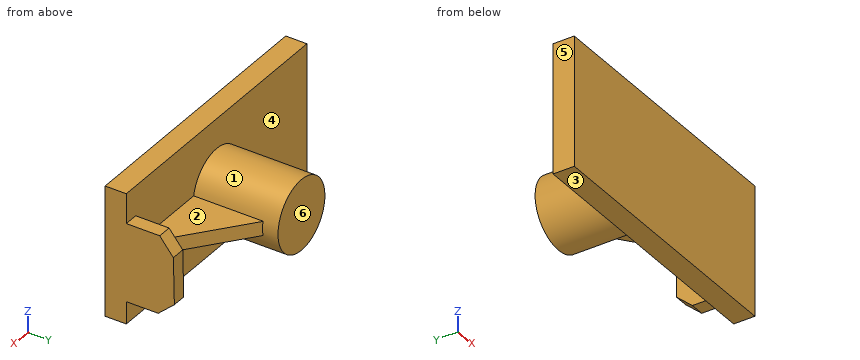
```python
from build123d import *

# Parameters (mm, degrees)
ESQUISSE1_W        = 192.615231554
ESQUISSE1_H        = 91.988888612
BOSS_EXTRU_1_DEPTH = 15
ESQUISSE3_R        = 25
BOSS_EXTRU_2_DEPTH = 60
BOSS_EXTRU_3_DEPTH = 10
NERVURE1_REACH     = 132.444
ESQUISSE5_WALL_W   = 340.670663134
ESQUISSE5_WALL_H   = 10


with BuildPart() as part:
    # Esquisse1 → Boss.-Extru.1 (new body)
    with BuildSketch(Plane(origin=(0, 0, 0), x_dir=(1, 0, 0), z_dir=(0, 1, 0))):
        Rectangle(ESQUISSE1_W, ESQUISSE1_H)
    extrude(amount=BOSS_EXTRU_1_DEPTH)

    # Esquisse3 → Boss.-Extru.2 (add)
    with BuildSketch(Plane(origin=(0, 15, 0), x_dir=(1, 0, 0), z_dir=(0, 1, 0))):
        with Locations(Location((0, 0, 0), (0, 0, 270))):
            Circle(ESQUISSE3_R)
    extrude(amount=BOSS_EXTRU_2_DEPTH)

    # Esquisse4 → Boss.-Extru.3 (add)
    with BuildSketch(Plane(origin=(96.307615777, 0, 0), x_dir=(0, 0, -1), z_dir=(1, 0, 0))):
        Polygon((-24.930682443, 15), (30.224142476, 15), (30.224142476, 37.550884027), (19.979617808, 48.99012657), (-12.997025488, 48.281884538), (-24.930682443, 38.617807381), align=None)
    extrude(amount=-BOSS_EXTRU_3_DEPTH)

    # Esquisse5 wall → Nervure1 (add, up to next)
    with BuildSketch(Plane(origin=(55.88995931, 39.234258268, 0), x_dir=(0.782119847954, -0.623128031336, 0), z_dir=(0.623128031336, 0.782119847954, 0)), mode=Mode.PRIVATE) as nervure1_sk1:
        Rectangle(ESQUISSE5_WALL_W, ESQUISSE5_WALL_H)
    nervure1_tool1 = extrude(nervure1_sk1.sketch, amount=-NERVURE1_REACH, mode=Mode.PRIVATE) - part.part
    add(nervure1_tool1.solids().sort_by_distance((55.88995931, 39.234258268, 0))[0])


solid = part.part
```
Here's how the part is built. I have some questions about the finished solid (model axes, mm). Face numbers are marked on the shaded views. A direction names the side the tool comes from. Round coordinates to 2 decimals unless told otherwise and drop trailing zeros. Write each loop counter-clockwise with the first axis right and the second up, starting at its lowest first coordinate (ties: lowest second). Pieces come first, ordered by that corner, then holes.
Q1. Please list where these lines run through material, in increasing order: probe 1 along Y at (x, z) = (-26, 8); probe 2 along X at (y, z) = (32, -30); probe 3 along X at (y, z) = (20.5, -1.5).
Q2. Which directions (+Z, -Z, +X, -X, +Y, -Y) give clear straight access to the entire face, cutting with the end or side of a thin tool? Please do the marked faces 1, 2 and 3.
Q3. If we section it at B-B on x = 0: Write out the boundary of the cut face in (y, z), plus the area to 3 significant figures.
Q4. If we section it at A-A on y = 45: Write out the boundary of the cut face in (x, z), plus the area to 3 significant figures.
Q5. If we section it at D-D on y = 26.5: Write out the boundary of the cut face in (x, z).
Q6. If we section it at C-C on z = -13.5: Write out the boundary of the cut face in (x, y), plus the area to 3 significant figures.
Q7. If we mould it in two halves opening along X, with no side actions, what happens to the marked faces 4, 5 and 6? For each: +X half, -X half, draft (parallel to the pull), parting line (faces both ways), or undercut.
Q8. Will these pins go through, and if not, where does the flat tip stop? P1, Ø2, axis at x = 6.5, y = 45.5, coming from the -Z side; P2, Ø5, axis at x = -49.5, z = 11, coming from the +Y side; P3, Ø3, axis at x = 0.5, z = -13, coming from the -Y side; P4, Ø5, axis at x = 91.5, y = 25, coming from the +Z side.
Answer below:
1. probe 1: y = 0 to 15
1. probe 2: x = 86.31 to 96.31
1. probe 3: x = -24.95 to 79.4, 86.31 to 96.31
2. face 1: +Y
2. face 2: +Z, +Y
2. face 3: -Z, +X, -X, +Y, -Y
3. outline: (0, -45.99) - (15, -45.99) - (15, -25) - (75, -25) - (75, 25) - (15, 25) - (15, 45.99) - (0, 45.99) - close
3. area: 4,380 mm2
4. outline: (24.49, -5) - (48.65, -5) - (48.65, 5) - (24.49, 5) arc R25 ccw (long way) to start; (86.31, -23.55) - (96.31, -23.55) - (96.31, 17.05) - (86.31, 17.05) - close
4. area: 2,610 mm2
5. outline: (24.49, -5) - (71.87, -5) - (71.87, 5) - (24.49, 5) arc R25 ccw (long way) to start; (86.31, -30.22) - (96.31, -30.22) - (96.31, 24.93) - (86.31, 24.93) - close
6. outline: (-96.31, 0) - (96.31, 0) - (96.31, 48.85) - (86.31, 48.85) - (86.31, 15) - (21.04, 15) - (21.04, 75) - (-21.04, 75) - (-21.04, 15) - (-96.31, 15) - close
6. area: 5,750 mm2
7. face 4: undercut
7. face 5: -X half
7. face 6: draft
8. P1: stops at z = -24.39
8. P2: stops at y = 15
8. P3: stops at y = 0
8. P4: stops at z = 24.93
